```python
from build123d import *


with BuildPart() as part:
    # Sweep1: sweep along a path in Sketch3
    with BuildLine(Plane(origin=(0, 6.039803803, 0), x_dir=(1, 0, 0), z_dir=(0, 1, 0))) as sweep1_path:
        Line((-25, 130), (25, 130))
        ThreePointArc((25, 130), (90, 65), (25, 0))
        Line((25, 0), (-25, 0))
        ThreePointArc((-25, 0), (-90, 65), (-25, 130))
    # Sketch1 → Sweep1 (sweep)
    with BuildSketch(Plane(origin=(0, 0, 0), x_dir=(0, 0, -1), z_dir=(1, 0, 0))):
        with BuildLine():
            Line((130.8, 8.039803803), (130, 8.039803803))
            Line((130, 8.039803803), (130, 6.039803803))
            Line((130, 6.039803803), (128.5, 6.039803803))
            ThreePointArc((128.5, 6.039803803), (134.474601817, -2.75615457), (129.150095427, -11.960196197))
            Line((129.150095427, -11.960196197), (131.150095427, -11.960196197))
            ThreePointArc((131.150095427, -11.960196197), (136.343285843, -1.866226416), (130.8, 8.039803803))
        make_face()
    sweep(path=sweep1_path.line)


solid = part.part
```
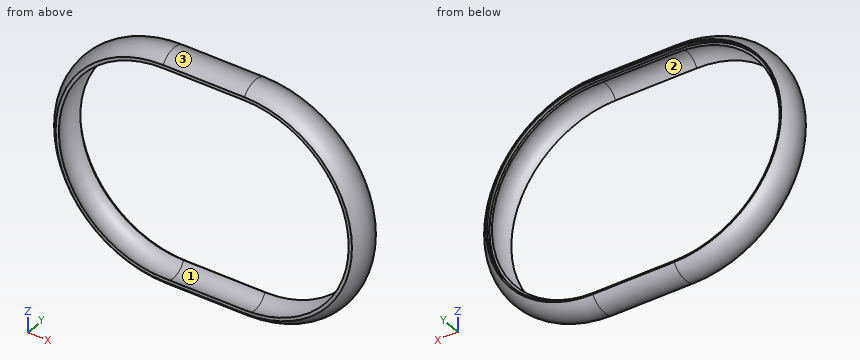
Here's how the part is built. I have some questions about the finished solid (model axes, mm). Face numbers are marked on the shaded views. Coordinates: 2 decimals unless noted, no trailing zeros. Order: outer loops, then holes, each group sorted by start corner. A loop starts at its lowest first (then second) coordinate and runs counter-clockwise, first axis right, second up.
Item 1: I need wall thicknesses on probe 1 along Z at (x, y) = (2, -1); probe 2 along X at (y, z) = (-7.75, -79); probe 3 along X at (y, z) = (4.5, -85). Which ranges of each line are inside material? Lowest first, please.
Response values:
probe 1: z = -136.3 to -134.25, 4.25 to 6.3
probe 2: x = -93.5 to -91.89, 91.89 to 93.5
probe 3: x = -91.44 to -87.86, 87.86 to 91.44
Item 2: Thinking about a two-plate mould opening in Y: for the marked faces 1, 2 and 3, which applies, pulls with the +Y half, pulls with the -Y half, needs draft (parallel to the pull), parting line crosses it, or undercut?
Response values:
face 1: undercut
face 2: undercut
face 3: parting line crosses it
Item 3: If we section it at A-A, the plane y = -5.5: List the corners of the cut face in (x, z) for me, then the cut area to 3 significant figures.
Response values:
outline: (-25, -135.85) - (25, -135.85) arc R70.85 ccw to (25, 5.85) - (-25, 5.85) arc R70.85 ccw to start; hole (-25, -134.19) - (25, -134.19) arc R69.19 ccw to (25, 4.19) - (-25, 4.19) arc R69.19 ccw to start
area: 893 mm2
Item 4: I'm going to push flat-ended pins straight in: pin 1 Ø8 at (y, z) = (-8.5, -64) entering from +X; pin 2 Ø0.6 at (x, y) = (-9, 7.5) entering from -Z; pin 3 Ø10 at (y, z) = (-8, -75.5) entering from -X. Where does each tip first touch, or does it pass through?
Response values:
pin 1: stops at x = 96.09
pin 2: stops at z = -131.96
pin 3: stops at x = -95.79
Item 5: If we section it at B-B, the plane z = -65: List the corners of the cut face in (x, y) for me.
Response values:
outline: (-91.15, -11.96) - (-89.15, -11.96) arc R10 cw to (-88.5, 6.04) - (-90, 6.04) - (-90, 8.04) - (-90.8, 8.04) arc R12 ccw to start; (88.5, 6.04) arc R10 cw to (89.15, -11.96) - (91.15, -11.96) arc R12 ccw to (90.8, 8.04) - (90, 8.04) - (90, 6.04) - close
